Can you work these out from the model? Positions are in its coordinate system, mm. A direction names the side the tool comes from. Round coordinates to 2 decimals unless told otherwise and drop trailing zeros. Loops run counter-clockwise (first coordinate to the right, second up) from the corner with the lowest first, then second, coordinate; pieces in that order, holes last. Notation, with made-up numbers: M -34.75,56.25 L 5.25,56.25 A24 cw 5.25,91.25 Z; hole C -31.75,-25.5 d6. An arc over 180 degrees is marked long. Return JSON: item names as keys, results as strings.
Autodesk Inventor part; units mm, degrees
ref_plane "YZ Plane" through (0, 0, 0) normal (1, 0, 0) x (0, 1, 0)
ref_plane "XZ Plane" through (0, 0, 0) normal (0, 1, 0) x (-1, 0, 0)
ref_plane "XY Plane" through (0, 0, 0) normal (0, 0, 1) x (1, 0, 0)
sketch "Sketch1" plane through (0, 0, 0) normal (0, 0, 1) x (1, 0, 0)
  line L0 (-32.4184, 42.5283) -> (-32.4184, -33.6717)
  line L1 (-32.4184, -33.6717) -> (43.7816, -33.6717)
  line L2 (43.7816, -33.6717) -> (43.7816, -33.4177)
  line L3 (37.6856, -27.3217) -> (-19.7184, -27.3217)
  line L4 (-26.0684, -20.9717) -> (-26.0684, 36.4323)
  line L5 (-32.1644, 42.5283) -> (-32.4184, 42.5283)
  arc A0 (-26.0684, 36.4323) -> (-32.1644, 42.5283) centre (-32.1644, 36.4323) ccw
  arc A1 (43.7816, -33.4177) -> (37.6856, -27.3217) centre (37.6856, -33.4177) ccw
  arc A2 (-26.0684, -20.9717) -> (-19.7184, -27.3217) centre (-19.7184, -20.9717) ccw
  dimension "d0" = 76.2
  dimension "d1" = 6.096
  dimension "d2" = 6.35
  dimension "d3" = 6.35
extrude "Extrusion1" add sketch "Sketch1" along normal blind 1828.8
properties part number "FE-00005-01"
Q1. I'm going to push flat-ended pins straight in: pin 1 Ø10 at (x, z) = (-22, 543.5) entering from +Y; pin 2 Ø2 at (x, z) = (0.5, 762.5) entering from +Y; pin 3 Ø3 at (y, z) = (-20, 211.5) entering from +X. Where does each tip first touch, or does it pass through?
Results:
{"pin 1": "stops at y = 39.67", "pin 2": "stops at y = -27.32", "pin 3": "stops at x = -26.05"}
Q2. On a 3-axis mill with a long thin cutter (end or side, diameter ignored), from which of +Z, -Z, +X, -X, +Y, -Y can I reach the whole of each face in a straight line? I mean faces 4 (the flat face through (9, -27.322, 902)), 5 (the flat face through (5, -33.672, 902)). Say none if no direction works.
Results:
{"face 4": "+Z, -Z, +X, +Y", "face 5": "+Z, -Z, +X, -X, -Y"}
Q3. Suppose I cut it at B-B, the plane y = -1. Please give me the cut outline in (x, z).
Results:
{"outline": "M -32.42,0 L -26.07,0 L -26.07,1828.8 L -32.42,1828.8 Z"}
Q4. If I drill on line 1 along X through (y, z) = (27, 747.5); line 2 along Y through (x, z) = (-12, 719.5); line 3 along X through (y, z) = (38, 1209), over which ranges is the centre line in solid material (lowest first)?
Results:
{"line 1": "x = -32.42 to -26.07", "line 2": "y = -33.67 to -27.32", "line 3": "x = -32.42 to -26.27"}
Q5. Thinking about a two-plate mould opening in X: for faces 1 (the flat face through (-26.068, 7, 902)), 2 (the flat face through (-28, -12, 0)), 3 (the flat face through (-32.418, 5, 902)), which applies, pulls with the +X half, pulls with the -X half, needs draft (parallel to the pull), parting line crosses it, or undercut?
Results:
{"face 1": "pulls with the +X half", "face 2": "needs draft", "face 3": "pulls with the -X half"}
Q6. Suppose I cut it at A-A, the plane x = 13.5. Please give me the cut outline in (y, z).
Results:
{"outline": "M -33.67,0 L -27.32,0 L -27.32,1828.8 L -33.67,1828.8 Z"}
